Geometry check sheet. Reference: the model listing, model coordinates, mm. A direction names the side the tool comes from. Round coordinates to 2 decimals unless told otherwise and drop trailing zeros. Order: outer loops, then holes, each group sorted by start corner. A loop starts at its lowest first (then second) coordinate and runs counter-clockwise, first axis right, second up. Notation, with made-up numbers: (66.5, -14) - (100.5, -14) arc R13 cw to (100.5, 10) - close; hole circle Ø5 at (9.25, 11.25). An arc over 180 degrees is marked (long way). One line per question, with ' | ' between items. Start each with the question number.
Q1. Sectioned sample at D-D, the plane x = 3.5. Enter the section's corners in (y, z), then the cut area to 3 significant figures.
Q2. Gauge pin test, flat ends, axial feed: P1, Ø4.5, axis at x = 7, y = 5.5, coming from the -Z side; P2, Ø2, axis at x = 7.5, z = -3.5, coming from the +Y side; P3, Ø6.5, axis at x = 6.5, y = 6, coming from the -Z side. Record the tip position at first contact, or that the pin passes through.
Q3. Sectioned sample at B-B, the plane x = 7. Enter the section's corners in (y, z).
Q4. Sectioned sample at A-A, the plane y = 5.5. Enter the section's corners in (x, z), then the cut area to 3 significant figures.
Q5. Material ranges on line 1 along Z through (x, y) = (3.95, -4.25); line 2 along Y through (x, z) = (8.25, 3); line 3 along Y through (x, z) = (9.25, 3), recorded low to high.
Q6. Tool access check on faces 1 (the face through (9, -5.5, -4)), 2 (the face through (8.94, -5.69, 0.05)), 3 (the face through (3.7, 5.3, 0)), 4 (the face through (1.27, -5.61, 0.61)). Record the directions out of +Z, -Z, +X, -X, +Y, -Y that give a thin tool (end or side, any length) a straight path to the whole face; none if there is none.
Q7. Sectioned sample at C-C, the plane z = 3.5. Enter the section's corners in (x, y), then the cut area to 3 significant figures.
Q8. Mould release check, pull along Z, two halves, no side actions. Record for faces 5 (the face through (8.94, -2.82, 0.03)), 6 (the face through (7, 0, 8)), 7 (the face through (4.07, 4.85, 2.46)): +Z half, -Z half, draft (parallel to the pull), parting line (faces both ways), or undercut.
```python
from build123d import *

# Parameters (mm, degrees)
BOSS_EXTRUDE1_DEPTH     = 13.5
SKETCH2_R               = 3
SKETCH2_W               = 11
SKETCH2_H               = 2.5
CUT_EXTRUDE1_DEPTH      = 9
CUT_EXTRUDE2_DEPTH      = 16.493950432
CUT_EXTRUDE2_DEPTH_BACK = 16.493950432
SKETCH3_R               = 1.75
CUT_EXTRUDE4_START      = -2.5
SKETCH4_R               = 1.75
CUT_EXTRUDE4_DEPTH      = 2.5
SKETCH5_R               = 1.75
CUT_EXTRUDE5_DEPTH      = 19.474644787
SKETCH6_R               = 3
SKETCH6_R_2             = 1.75
CUT_EXTRUDE6_DEPTH      = 5
FILLET1_R               = 3
FILLET2_R               = 2


with BuildPart() as part:
    # Sketch1 → Boss-Extrude1 (new body)
    with BuildSketch(Plane(origin=(0, 0, 0), x_dir=(0, 0, -1), z_dir=(1, 0, 0))):
        Polygon((-8, 9.75), (-8, -9.75), (8, -9.75), (8, 1), (0, 1), (0, 9.75), align=None)
    extrude(amount=BOSS_EXTRUDE1_DEPTH)

    # Sketch2 → Cut-Extrude1 (cut)
    with BuildSketch(Plane(origin=(13.5, 0, 0), x_dir=(0, 0, -1), z_dir=(1, 0, 0))):
        with Locations((-3, -4.25)):
            Circle(SKETCH2_R)
        with Locations((2.5, -4.25)):
            Rectangle(SKETCH2_W, SKETCH2_H)
    extrude(amount=-CUT_EXTRUDE1_DEPTH, mode=Mode.SUBTRACT)

    # Sketch3 → Cut-Extrude2 (cut, two sides: drawn at the far end of the back side and taken through both)
    with BuildSketch(Plane(origin=(4.5, 0, 0), x_dir=(0, 0, -1), z_dir=(1, 0, 0)).offset(-CUT_EXTRUDE2_DEPTH_BACK)):
        with Locations((-3, -4.25)):
            Circle(SKETCH3_R)
    extrude(amount=CUT_EXTRUDE2_DEPTH + CUT_EXTRUDE2_DEPTH_BACK, mode=Mode.SUBTRACT)

    # Sketch4 → Cut-Extrude4 (cut)
    with BuildSketch(Plane.ZY.offset(CUT_EXTRUDE4_START)):
        Polygon((6.175426481, -4.25), (4.58771324, -1.5), (1.41228676, -1.5), (-0.175426481, -4.25), (1.41228676, -7), (4.58771324, -7), align=None)
        with Locations(Location((3, -4.25, 0), (0, 0, 180))):
            Circle(SKETCH4_R, mode=Mode.SUBTRACT)
    extrude(amount=CUT_EXTRUDE4_DEPTH, mode=Mode.SUBTRACT)

    # Sketch5 → Cut-Extrude5 (cut, through all)
    with BuildSketch(Plane(origin=(0, 0, 0), x_dir=(-1, 0, 0), z_dir=(0, 0, -1))):
        with Locations(Location((-7, 5.5, 0), (0, 0, 90))):
            Circle(SKETCH5_R)
    extrude(amount=-CUT_EXTRUDE5_DEPTH, mode=Mode.SUBTRACT)

    # Sketch6 → Cut-Extrude6 (cut)
    with BuildSketch(Plane(origin=(0, 0, 0), x_dir=(-1, 0, 0), z_dir=(0, 0, -1))):
        with Locations(Location((-7, 5.5, 0), (0, 0, 90))):
            Circle(SKETCH6_R)
        with Locations(Location((-7, 5.5, 0), (0, 0, 90))):
            Circle(SKETCH6_R_2, mode=Mode.SUBTRACT)
    extrude(amount=-CUT_EXTRUDE6_DEPTH, mode=Mode.SUBTRACT)

    # Fillet1
    fillet1_edges = [part.edges().sort_by_distance(p)[0] for p in [
        (13.5, 9.75, 4),
    ]]
    fillet(fillet1_edges, radius=FILLET1_R)

    # Fillet2
    fillet2_edges = [part.edges().sort_by_distance(p)[0] for p in [
        (9, -3, 0.272821971),
        (9, -5.5, 0.272821971),
    ]]
    fillet(fillet2_edges, radius=FILLET2_R)


solid = part.part
```
Determined:
1) outline: (-9.75, -8) - (1, -8) - (1, 0) - (9.75, 0) - (9.75, 8) - (-9.75, 8) - close; hole circle Ø3.5 at (-4.25, 3) | area: 232 mm2
2) P1: stops at z = 5 | P2: stops at y = 1 | P3: stops at z = 0
3) outline: (-9.75, -8) - (-5.5, -8) - (-5.5, -0.8) arc R2 ccw to (-6.2, 0.72) arc R3 cw (long way) to (-2.3, 0.72) arc R2 ccw to (-3, -0.8) - (-3, -8) - (1, -8) - (1, 0) - (2.5, 0) - (2.5, 5) - (3.75, 5) - (3.75, 8) - (-9.75, 8) - close; (7.25, 5) - (8.5, 5) - (8.5, 0) - (9.75, 0) - (9.75, 8) - (7.25, 8) - close
4) outline: (0, 0) - (4, 0) - (4, 5) - (5.25, 5) - (5.25, 8) - (0, 8) - close; (8.75, 5) - (10, 5) - (10, 0) - (13.5, 0) - (13.5, 8) - (8.75, 8) - close | area: 67.5 mm2
5) line 1: z = -8 to 1.25, 4.75 to 8 | line 2: y = -9.75 to -7.25, -1.25 to 2.77, 8.23 to 9.75 | line 3: y = -9.75 to -7.25, -1.25 to 3.52, 7.48 to 9.75
6) face 1: -Z, +X | face 2: +X | face 3: -Z, +X, -X, +Y | face 4: -X
7) outline: (0, -9.75) - (13.5, -9.75) - (13.5, -7.21) - (4.5, -7.21) - (4.5, -5.93) - (2.5, -5.93) - (2.5, -7) - (0, -7) - close; (0, -1.5) - (2.5, -1.5) - (2.5, -2.57) - (4.5, -2.57) - (4.5, -1.29) - (13.5, -1.29) - (13.5, 6.75) arc R3 ccw to (10.5, 9.75) - (0, 9.75) - close; hole circle Ø6 at (7, 5.5) | area: 159 mm2
8) face 5: undercut | face 6: +Z half | face 7: draft
